```python
from build123d import *

# Parameters (mm, degrees)
PAD015_DEPTH                        = 3
SKETCH054_R                         = 1.7
POCKET018_DEPTH                     = 0.001
POCKET018_DEPTH_BACK                = 3.001
BODY001003005003004_PLACEMENT_ANGLE = 60
CLONE022_PLACEMENT_ANGLE            = 32


with BuildPart() as part:
    # Sketch053 → Pad015 (new body)
    with BuildSketch(Plane.XY):
        with BuildLine():
            Line((0, 182.848457), (0, 197.848457))
            ThreePointArc((141.077868, 138.712102), (76.485413, 182.466418), (0, 197.848457))
            ThreePointArc((141.062279, 137.294387), (141.364747, 138.000004), (141.077868, 138.712102))
            Line((131.746186, 128.227134), (141.062279, 137.294387))
            ThreePointArc((130.335906, 128.242388), (131.037899, 127.943805), (131.746186, 128.227134))
            ThreePointArc((130.335906, 128.242388), (70.656336, 168.64531), (0, 182.848457))
        make_face()
    pad015 = extrude(amount=PAD015_DEPTH)

    # Mirrored020: Pad015 across Sketch053 V_Axis
    add(pad015.mirror(Plane(origin=(0, 0, 0), x_dir=(0, 0, 1), z_dir=(1, 0, 0))))

    # Sketch054 → Pocket018 (cut, two sides)
    with BuildSketch(Plane.XY) as pocket018_sk:
        with Locations((129.243686, 139.741203)):
            Circle(SKETCH054_R)
        with Locations((0, 190.345828)):
            Circle(SKETCH054_R)
        with Locations((-129.243686, 139.741203)):
            Circle(SKETCH054_R)
    extrude(amount=-POCKET018_DEPTH, mode=Mode.SUBTRACT)
    extrude(pocket018_sk.sketch, amount=POCKET018_DEPTH_BACK, mode=Mode.SUBTRACT)


with BuildPart() as part_1:
    # Body001003005003004 placement: moved
    add(part.part.rotate(Axis((0, 0, 0), (0, 0, 1)), BODY001003005003004_PLACEMENT_ANGLE))


with BuildPart() as part_2:
    # Clone022 placement: moved
    add(part_1.part.moved(Location((388, 926, 0))).rotate(Axis((388, 926, 0), (0, 0, 1)), CLONE022_PLACEMENT_ANGLE))


solid = part_2.part
```
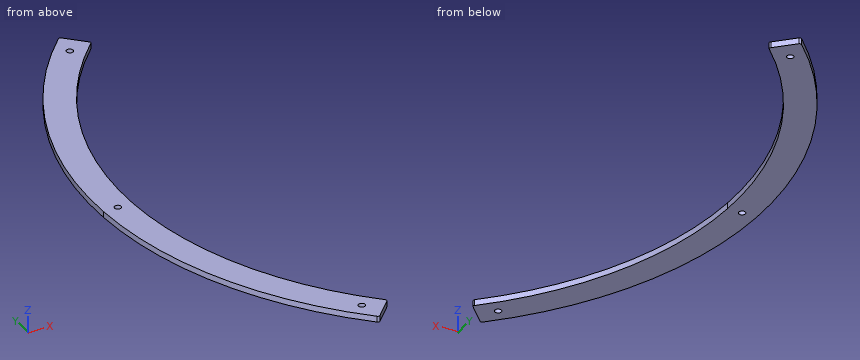
Source: CAD feature listing. Evaluate the final solid. Frame: model axes, mm. Round coordinates to 2 decimals unless told otherwise and drop trailing zeros. Loops run counter-clockwise (first coordinate to the right, second up) from the corner with the lowest first, then second, coordinate; pieces in that order, holes last. Notation, with made-up numbers: M 19,-40 L 31,-40 A26 ccw 31,-9 Z; hole C 36.5,28.5 d2. An arc over 180 degrees is marked long. Put each result on its own line as item: value.
(1) Section D-D, the plane y = 1028.5. Return loops of the section in (x, z).
Solutions:
outline: M 218.77,0 L 236.58,0 L 236.58,3 L 218.77,3 Z
(2) Section A-A, the plane x = 220.5. Return loops of the section in (y, z).
Solutions:
outline: M 820.7,0 L 852.67,0 L 852.67,3 L 820.7,3 Z; M 999.33,0 L 1031.3,0 L 1031.3,3 L 999.33,3 Z
(3) Section B-B, the plane z = 0.5. Return loops of the section in (x, y).
Solutions:
outline: M 190.27,919.1 A197.85 ccw 254.3,780.17 A1 ccw 255.71,780.23 L 264.45,789.86 A1 ccw 264.38,791.27 A182.85 cw 205.26,919.62 A182.85 cw 255.29,1051.78 A1 ccw 255.25,1053.19 L 245.87,1062.18 A1 ccw 244.45,1062.15 A197.85 ccw Z; hole C 197.77,919.36 d3.4; hole C 243.83,1050.29 d3.4; hole C 252.85,791.96 d3.4
(4) Section C-C, the plane y = 824.5. Return loops of the section in (x, z).
Solutions:
outline: M 218.17,0 L 235.91,0 L 235.91,3 L 218.17,3 Z
(5) Ray query, line 1 (Y direction, x = 239, z = 1.05); line 2 (Y direction, x = 225, z = 0.8); line 3 (X direction, y = 928, z = 2.3). Return the intervals inside material, ascending. Write a range as [from, to].
Solutions:
line 1: [795.83, 820.02], [1031.98, 1056.17]
line 2: [813.86, 843.15], [1008.85, 1038.14]
line 3: [190.16, 205.16]
